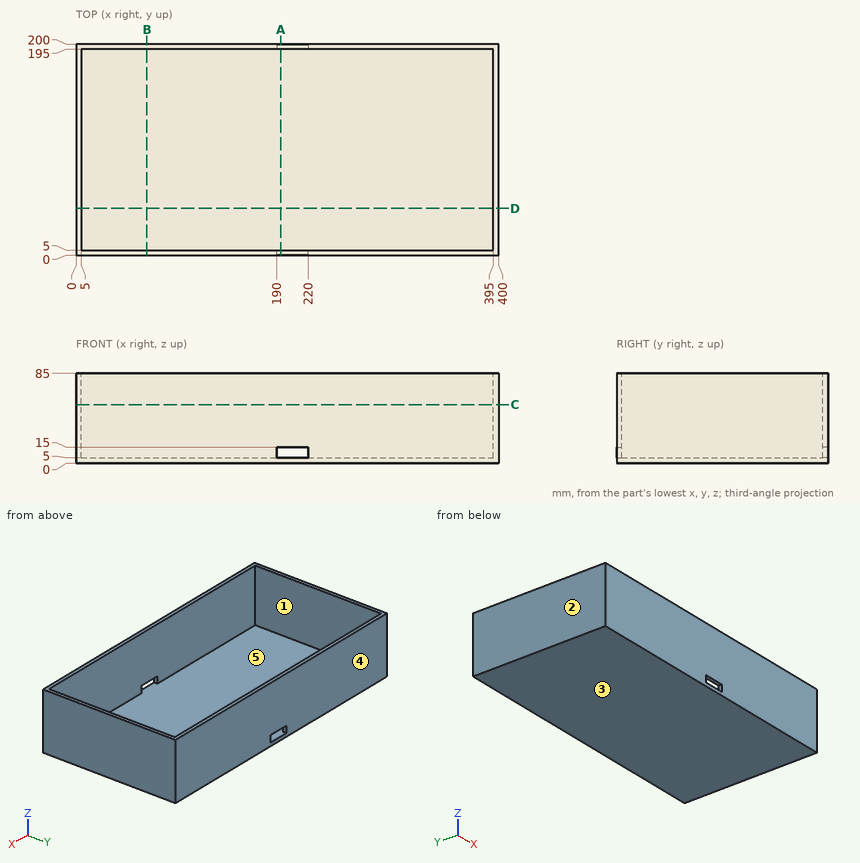
Here's the drawing with two shaded views (mm, measured from the low corner). I have some questions. A direction names the side the tool comes from. Coordinates: 2 decimals unless noted, no trailing zeros. Write each loop counter-clockwise with the first axis right and the second up, starting at its lowest first coordinate (ties: lowest second). Pieces come first, ordered by that corner, then holes. Notation, with made-up numbers: M -39,11 L -24,11 A12 ccw -24,21 Z; hole C 58.25,-38 d6. An arc over 180 degrees is marked long. Answer as CSV lines item,"result".
Item 1: I'm going to push flat-ended pins straight in: P1, Ø10, axis at x = 354.5, z = 24, coming from the -Y side; P2, Ø1.5, axis at x = 333, y = 111, coming from the +Z side. Where does each tip first touch, or does it pass through?
Geometry results:
P1,"stops at y = 0"
P2,"stops at z = 5"
Item 2: Imagine slicing it at C-C on z = 55.5. List the corners of the cut face in (x, y) for me.
Geometry results:
outline,"M 0,0 L 400,0 L 400,200 L 0,200 Z; hole M 5,5 L 395,5 L 395,195 L 5,195 Z"
Item 3: Please list where these lines run through material, in increasing order: line 1 along Y through (x, z) = (172.5, 30); line 2 along X through (y, z) = (55.5, 12); line 3 along Z through (x, y) = (189, 62).
Geometry results:
line 1,"y = 0 to 5, 195 to 200"
line 2,"x = 0 to 5, 395 to 400"
line 3,"z = 0 to 5"
Item 4: We'd pull the mould along Y, two halves only. Please class the marked faces 3, 4 and 5: +Y half, -Y half, draft (parallel to the pull), parting line (faces both ways), or undercut.
Geometry results:
face 3,"draft"
face 4,"+Y half"
face 5,"undercut"
Item 5: Imagine slicing it at D-D on y = 44.5. List the corners of the cut face in (x, z) for me, plus the area to 3 significant figures.
Geometry results:
outline,"M 0,0 L 400,0 L 400,85 L 395,85 L 395,5 L 5,5 L 5,85 L 0,85 Z"
area,"2,800 mm2"
Item 6: Imagine slicing it at B-B on x = 67. List the corners of the cut face in (y, z) for me.
Geometry results:
outline,"M 0,0 L 200,0 L 200,85 L 195,85 L 195,5 L 5,5 L 5,85 L 0,85 Z"
Item 7: Imagine slicing it at A-A on x = 194. List the corners of the cut face in (y, z) for me, plus the area to 3 significant figures.
Geometry results:
outline,"M 0,0 L 200,0 L 200,5 L 0,5 Z; M 0,15 L 5,15 L 5,85 L 0,85 Z; M 195,15 L 200,15 L 200,85 L 195,85 Z"
area,"1,700 mm2"
Item 8: On a 3-axis mill with a long thin cutter (end or side, diameter ignored), from which of +Z, -Z, +X, -X, +Y, -Y can I reach the whole of each face in a straight line? I mean the marked faces 1 and 2. Say none if no direction works.
Geometry results:
face 1,"+Z"
face 2,"+Z, -Z, -X, +Y, -Y"
